from build123d import *

# Parameters (mm, degrees)
F0_R     = 16
F0_R_2   = 1.5875
F1_DEPTH = 6.75
F2_R     = 4.7625
F2_R_2   = 1.5875
F3_DEPTH = 11.500002
F4_R     = 1.5875


with BuildPart() as f1:
    # F0 (on Top) → F1 (new body, symmetric)
    with BuildSketch(Plane.XY):
        Circle(F0_R)
        Circle(F0_R_2, mode=Mode.SUBTRACT)
    extrude(amount=F1_DEPTH, both=True)

    # F2 (on Top) → F3 (join, symmetric)
    with BuildSketch(Plane.XY):
        Circle(F2_R)
        Circle(F2_R_2, mode=Mode.SUBTRACT)
    extrude(amount=F3_DEPTH, both=True)

    # F4
    f4_edges = [f1.edges().sort_by_distance(p)[0] for p in [
        (-16, 0, 6.75),
        (-16, 0, -6.75),
    ]]
    fillet(f4_edges, radius=F4_R)


solid = f1.part
Source: CAD feature listing. Evaluate the final solid. Frame: model axes, mm. A direction names the side the tool comes from. Coordinates: 2 decimals unless noted, no trailing zeros. Loops run counter-clockwise (first coordinate to the right, second up) from the corner with the lowest first, then second, coordinate; pieces in that order, holes last. Notation, with made-up numbers: M 12.25,61.5 L 59.25,61.5 A19 ccw 59.25,91.5 Z; hole C -31,-21.75 d3. An arc over 180 degrees is marked long. Answer in a Markdown table with one row per item.
Q1. Set-up query: faces 4 (the flat face through (6, 0, 6.75)), 5 (the flat face through (6, 0, -6.75)), 6 (the cylindrical face through (-3.47, -15.62, 0.07)). Return all of +Z, -Z, +X, -X, +Y, -Y with unobstructed straight access to the full face (end or side cutting, diameter ignored); none if empty.
Answers below:
| item | result |
|---|---|
| face 4 | +Z |
| face 5 | -Z |
| face 6 | +Z, -Z |
Q2. Section D-D on z = 4.75. Return the cut outline in (x, y) (1 decimal), plus the area to 3 significant figures.
Answers below:
| item | result |
|---|---|
| outline | C 0,0 d32; hole C 0,0 d3.2 |
| area | 796 mm^2 |
Q3. Section C-C on z = -9.5. Return the cut outline in (x, y) (1 decimal).
Answers below:
| item | result |
|---|---|
| outline | C 0,0 d9.5; hole C 0,0 d3.2 |
Q4. First-contact query: pin 1 (6 mm diameter, centred on y = -12, z = 1.5, fed in from +X); pin 2 (10 mm diameter, centred on x = 5.5, z = 5.5, fed in from +Y); pin 3 (3 mm diameter, centred on y = -9, z = -3, fed in from -X). Flat tips, straight axial feed; report the tip coordinate or a pass-through.
Answers below:
| item | result |
|---|---|
| pin 1 | stops at x = 13.23 |
| pin 2 | stops at y = 15.99 |
| pin 3 | stops at x = -14.13 |
Q5. Draft query along Y for faces 1 (the cylindrical face through (-3.78, -2.9, -9.09)), 2 (the flat face through (2, 0, -11.5)), 3 (the cylindrical face through (-0.34, -1.55, -0.16)). Return one class per face: pulls with the +Y half, pulls with the -Y half, needs draft (parallel to the pull), parting line crosses it, or undercut.
Answers below:
| item | result |
|---|---|
| face 1 | parting line crosses it |
| face 2 | needs draft |
| face 3 | undercut |
Q6. Ray query, probe 1 along Y at (x, z) = (0, -3.5); probe 2 along Z at (x, y) = (-2, -10); probe 3 along X at (y, z) = (0.5, -0.75). Return the intervals inside material, ascending. Write a range as from..to.
Answers below:
| item | result |
|---|---|
| probe 1 | y = -16..-1.59, 1.59..16 |
| probe 2 | z = -6.75..6.75 |
| probe 3 | x = -15.99..-1.51, 1.51..15.99 |
